from build123d import *

# Parameters (mm, degrees)
F0_R      = 30.5
F1_DEPTH  = 3
F3_DEPTH  = 80
F4_R      = 23.49999
F5_W      = 10
F5_H      = 10
F6_DEPTH  = 10
F7_SIZE   = 9.99999
F8_W      = 10
F8_H      = 10
F9_DEPTH  = 10
F10_SIZE  = 9.99999
F11_R     = 5
F12_DEPTH = 3
F13_R     = 5
F14_DEPTH = 3


# Not quite as in the source:
# - a fillet or chamfer is up to 0.001 mm smaller than in the source, because OpenCascade refuses the exact size


with BuildPart() as f1:
    # F0 (on Top) → F1 (new body)
    with BuildSketch(Plane.XY):
        Circle(F0_R)
    extrude(amount=F1_DEPTH)

    # F2 (on face) → F3 (join)
    with BuildSketch(Plane.XY.offset(3)):
        Polygon((1.5, 23.5), (0, 23.5), (-1.5, 23.5), (-1.5, 0), (-1.5, -23.5), (0, -23.5), (1.5, -23.5), (1.5, 0), align=None)
    extrude(amount=F3_DEPTH)

    # F4 (radius 23.5 in the source; OpenCascade refuses exactly that, so slightly less here)
    f4_edges = [f1.edges().sort_by_distance(p)[0] for p in [
        (0, 23.5, 83),
        (0, -23.5, 83),
    ]]
    fillet(f4_edges, radius=F4_R)

    # F5 (on face) → F6 (join)
    with BuildSketch(Plane.XY.offset(3)):
        with Locations((6.5, -18.5)):
            Rectangle(F5_W, F5_H)
    extrude(amount=F6_DEPTH)

    # F7 (size 10 in the source; OpenCascade refuses exactly that, so slightly less here)
    f7_edges = [f1.edges().sort_by_distance(p)[0] for p in [
        (11.5, -18.5, 13),
    ]]
    chamfer(f7_edges, length=F7_SIZE)

    # F8 (on face) → F9 (join)
    with BuildSketch(Plane.XY.offset(3)):
        with Locations((6.5, 18.5)):
            Rectangle(F8_W, F8_H)
        with Locations((-6.5, 18.5)):
            Rectangle(F8_W, F8_H)
        with Locations((-6.5, -18.5)):
            Rectangle(F8_W, F8_H)
    extrude(amount=F9_DEPTH)

    # F10 (size 10 in the source; OpenCascade refuses exactly that, so slightly less here)
    f10_edges = [f1.edges().sort_by_distance(p)[0] for p in [
        (11.5, 18.5, 13),
        (-11.5, 18.5, 13),
        (-11.5, -18.5, 13),
    ]]
    chamfer(f10_edges, length=F10_SIZE)

    # F11 (on face) → F12 (cut)
    with BuildSketch(Plane.XY.offset(3)):
        with BuildLine():
            ThreePointArc((21.5, 0), (16.5, 5), (11.5, 0))
            ThreePointArc((11.5, 0), (16.5, -5), (21.5, 0))
        make_face()
        with Locations((-16.5, 0)):
            Circle(F11_R)
    extrude(amount=-F12_DEPTH, mode=Mode.SUBTRACT)

    # F13 (on face) → F14 (cut)
    with BuildSketch(Plane.YZ.offset(1.5)):
        with BuildLine():
            ThreePointArc((0, 77.6050660014), (-5, 72.6050660014), (0, 67.6050660014))
            ThreePointArc((0, 67.6050660014), (3.5355339059, 69.0695320955), (5, 72.6050660014))
            ThreePointArc((5, 72.6050660014), (3.5355339059, 76.1405999073), (0, 77.6050660014))
        make_face()
        with Locations((11.75, 57.0152029395)):
            Circle(F13_R)
        with BuildLine():
            ThreePointArc((0, 48), (-5, 43), (0, 38))
            ThreePointArc((0, 38), (3.5355339059, 39.4644660941), (5, 43))
            ThreePointArc((5, 43), (3.5355339059, 46.5355339059), (0, 48))
        make_face()
        with Locations((-11.75, 57.0152029395)):
            Circle(F13_R)
        with Locations((-11.75, 25.4681762308)):
            Circle(F13_R)
        with Locations((11.75, 25.4681762308)):
            Circle(F13_R)
    extrude(amount=-F14_DEPTH, mode=Mode.SUBTRACT)


solid = f1.part
Check sheet for the modelled part. Datum: model origin and axes. Units: mm. A direction names the side the tool comes from. Round coordinates to 2 decimals unless told otherwise and drop trailing zeros. Loops run counter-clockwise (first coordinate to the right, second up) from the corner with the lowest first, then second, coordinate; pieces in that order, holes last. Notation, with made-up numbers: (-16, 55) -> (37, 55) arc R18 cw to (37, 66) -> close; hole circle Ø6 at (13.25, 15). An arc over 180 degrees is marked (long way). Put each result on its own line as item: value. Start each with the question number.
1. Draft check along X on faces 1 (the face through (-21.495, 0.22, 1.521)), 2 (the face through (0.02, -16.8, 75.93)), 3 (the face through (6.6, 18.4, 7.9)), 4 (the face through (21.495, -0.22, 1.521)). Enter one of: +X half, -X half, draft (parallel to the pull), parting line (faces both ways), or undercut.
2. Section check B-B (x = -17.5). Enter the section's corners in (y, z), plus the area to 3 significant figures.
3. Section check A-A (y = 11.75). Enter the section's corners in (x, z).
4. Gauge pin test, flat ends, axial feed: pin 1 (12 mm diameter, centred on x = 1.5, z = 46, fed in from +Y); pin 2 (9 mm diameter, centred on y = -11.75, z = 57.02, fed in from -X); pin 3 (3 mm diameter, centred on y = 9, z = 67.5, fed in from -X); pin 4 (11 mm diameter, centred on x = 4.5, z = 7.5, fed in from +Y). Record the tip position at first contact, or that the pin passes through.
5. Section check C-C (z = 45.5). Enter the section's corners in (x, y), plus the area to 3 significant figures.
6. Section check D-D (y = -1). Enter the section's corners in (x, z), plus the area to 3 significant figures.
7. Scan lines: probe 1 along Z at (x, y) = (0, -11); probe 2 along Z at (x, y) = (-0.75, -11.75); probe 3 along X at (y, z) = (-23, 26). Record each from-to range of solid material in increasing order.
8. Access from +Z, -Z, +X, -X, +Y, -Y to the whole of each face (thin tool, end or side, straight path). Record for faces 5 (the face through (-5, -13.5, 7)), 6 (the face through (6, 0, 3)), 7 (the face through (5, 13.5, 7)), 8 (the face through (-1, -23.5, 21)).
Findings:
1. face 1: undercut
1. face 2: draft
1. face 3: +X half
1. face 4: undercut
2. outline: (-24.98, 0) -> (-4.9, 0) -> (-4.9, 3) -> (-24.98, 3) -> close; (4.9, 0) -> (24.98, 0) -> (24.98, 3) -> (4.9, 3) -> close
2. area: 120 mm^2
3. outline: (-28.15, 0) -> (28.15, 0) -> (28.15, 3) -> (1.5, 3) -> (1.5, 20.47) -> (-1.5, 20.47) -> (-1.5, 3) -> (-28.15, 3) -> close; (-1.5, 30.47) -> (1.5, 30.47) -> (1.5, 52.02) -> (-1.5, 52.02) -> close; (-1.5, 62.02) -> (1.5, 62.02) -> (1.5, 79.85) -> (-1.5, 79.85) -> close
4. pin 1: stops at y = 23.5
4. pin 2: passes through
4. pin 3: stops at x = -1.5
4. pin 4: stops at y = 30.47
5. outline: (-1.5, -23.5) -> (1.5, -23.5) -> (1.5, -4.33) -> (-1.5, -4.33) -> close; (-1.5, 4.33) -> (1.5, 4.33) -> (1.5, 23.5) -> (-1.5, 23.5) -> close
5. area: 115 mm^2
6. outline: (-30.48, 0) -> (-21.4, 0) -> (-21.4, 3) -> (-30.48, 3) -> close; (-11.6, 0) -> (11.6, 0) -> (11.6, 3) -> (1.5, 3) -> (1.5, 38.1) -> (-1.5, 38.1) -> (-1.5, 3) -> (-11.6, 3) -> close; (-1.5, 47.9) -> (1.5, 47.9) -> (1.5, 67.71) -> (-1.5, 67.71) -> close; (-1.5, 77.5) -> (1.5, 77.5) -> (1.5, 82.98) -> (-1.5, 82.98) -> close; (21.4, 0) -> (30.48, 0) -> (30.48, 3) -> (21.4, 3) -> close
6. area: 305 mm^2
7. probe 1: z = 0 to 20.52, 30.41 to 52.07, 61.96 to 80.27
7. probe 2: z = 0 to 20.47, 30.47 to 52.02, 62.02 to 79.85
7. probe 3: x = -1.5 to 1.5
8. face 5: +Z, -X
8. face 6: +Z
8. face 7: +Z, +X
8. face 8: +Z, +X, -X, -Y
